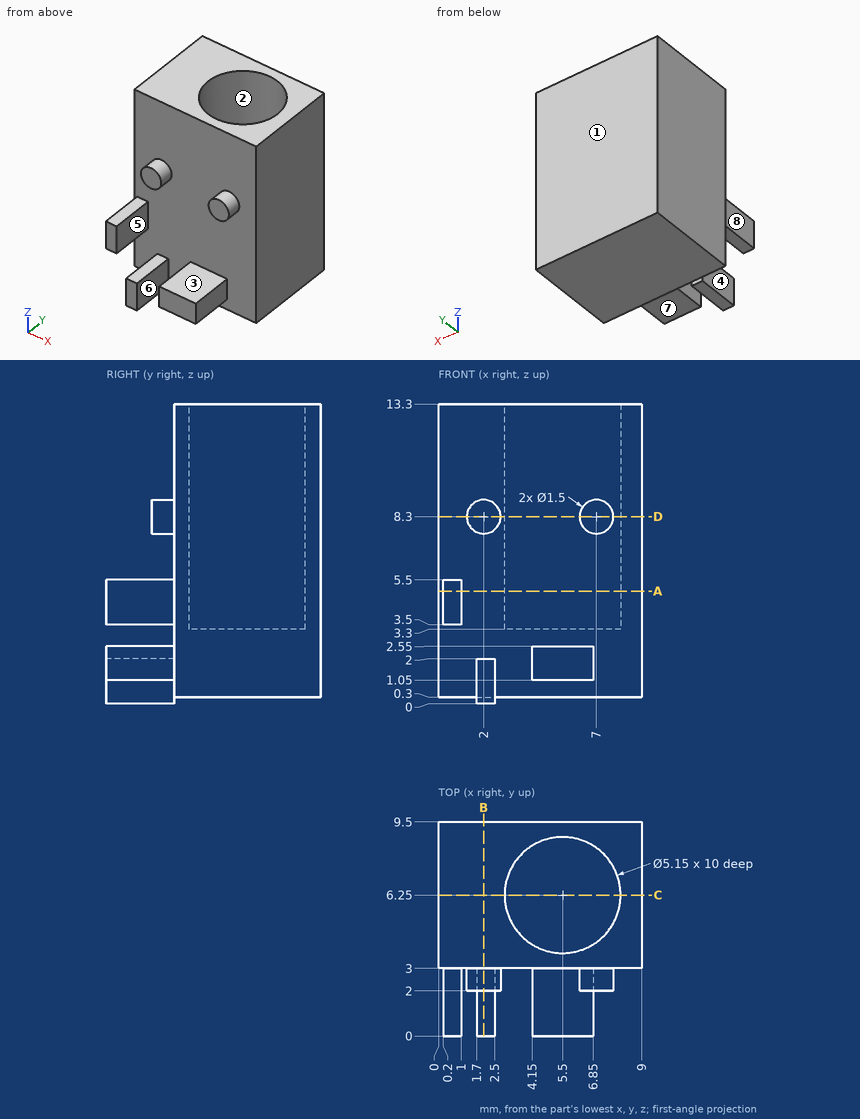
Study the drawing (mm; zero at the part's minimum x, y, z) and answer. A direction names the side the tool comes from. Round coordinates to 2 decimals unless told otherwise and drop trailing zeros. Loops run counter-clockwise (first coordinate to the right, second up) from the corner with the lowest first, then second, coordinate; pieces in that order, holes last. Notation, with made-up numbers: (18, 68.25) - (65, 68.25) arc R14 ccw to (65, 86.25) - close; hole circle Ø3 at (27.25, 66.25). An arc over 180 degrees is marked (long way). Use one line per item in the form item = value. Start each with the question number.
1. Consider line 1 (Y direction, x = 5.5, z = 10.5) (3 decimals); line 2 (Y direction, x = 2, z = 7.5); line 3 (X direction, y = 4.25, z = 12). Determine where each line is inside the solid, lowest interval first. Write a range as [from, to].
2. A tool of negligible diameter and unlimited length cuts with its end or side. For the marked faces 4, 5, 6, 7 and 8, from which of +Z, -Z, +X, -X, +Y, -Y can it reach the whole face along a straight path? Write none if from no direction.
3. Given pin 1 Ø3 at (x, y) = (5.5, 6.25) entering from -Z; pin 2 Ø0.8 at (x, y) = (5, 1) entering from +Z; pin 3 Ø0.8 at (x, z) = (7, 8.5) entering from -Y; pin 4 Ø4 at (y, z) = (6, 5.5) entering from -X, each flat-ended and moving along its own axis, determine where each tip first touches the part or whether it passes through.
4. The part is cut by section A-A on z = 5. Determine the outline of the cut face in (x, y) (3 decimals).
5. The part is cut by section D-D on z = 8.3. Determine the outline of the cut face in (x, y) (3 decimals).
6. The part is cut by section C-C on y = 6.25. Determine the outline of the cut face in (x, z) (3 decimals).
7. The part is cut by section B-B on x = 2. Determine the outline of the cut face in (y, z).
8. For a pull along Y with two mould halves and no side action, classify the marked faces 1, 2 and 3 as pulls with the +Y half, pulls with the -Y half, needs draft (parallel to the pull), parting line crosses it, or undercut.
Geometry check:
q1.line_1 = [3, 3.675], [8.825, 9.5]
q1.line_2 = [3, 9.5]
q1.line_3 = [0, 3.88], [7.12, 9]
q2.face_4 = -Z, -X, -Y
q2.face_5 = +Z, -Z, +X, -Y
q2.face_6 = -Z, -Y
q2.face_7 = -Z, +X, -Y
q2.face_8 = +Z, -Z, -X, -Y
q3.pin_1 = 0.3
q3.pin_2 = 2.55
q3.pin_3 = 2
q3.pin_4 = 0
q4.outline = (0, 3) - (0.2, 3) - (0.2, 0) - (1, 0) - (1, 3) - (9, 3) - (9, 9.5) - (0, 9.5) - close; hole circle Ø5.15 at (5.5, 6.25)
q5.outline = (0, 3) - (1.25, 3) - (1.25, 2) - (2.75, 2) - (2.75, 3) - (6.25, 3) - (6.25, 2) - (7.75, 2) - (7.75, 3) - (9, 3) - (9, 9.5) - (0, 9.5) - close; hole circle Ø5.15 at (5.5, 6.25)
q6.outline = (0, 0.3) - (9, 0.3) - (9, 13.3) - (8.075, 13.3) - (8.075, 3.3) - (2.925, 3.3) - (2.925, 13.3) - (0, 13.3) - close
q7.outline = (0, 0) - (3, 0) - (3, 0.3) - (9.5, 0.3) - (9.5, 13.3) - (3, 13.3) - (3, 9.05) - (2, 9.05) - (2, 7.55) - (3, 7.55) - (3, 2) - (0, 2) - close
q8.face_1 = pulls with the +Y half
q8.face_2 = undercut
q8.face_3 = needs draft
